Read the model definition and answer for the solid it produces. Units are mm, in the model's axes. A direction names the side the tool comes from. Coordinates: 2 decimals unless noted, no trailing zeros. Loops run counter-clockwise (first coordinate to the right, second up) from the corner with the lowest first, then second, coordinate; pieces in that order, holes last. Notation, with made-up numbers: (83, 10.5) -> (111, 10.5) arc R21 ccw to (111, 23.5) -> close; hole circle Ø11 at (49, 89). An arc over 180 degrees is marked (long way). Answer as CSV lines item,"result".
```python
from build123d import *

# Parameters (mm, degrees)
F0_W     = 5
F0_H     = 3
F1_DEPTH = 5
F2_DEPTH = 23


with BuildPart() as f1:
    # F0 (on Top) → F1 (new body)
    with BuildSketch(Plane.XY):
        Rectangle(F0_W, F0_H)
        with BuildLine():
            ThreePointArc((-0.5, 0.5), (0, 1), (0.5, 0.5))
            Line((0.5, 0.5), (1.27, 0.5))
            ThreePointArc((1.27, 0.5), (1.6235533906, 0.3535533906), (1.77, 0))
            ThreePointArc((1.77, 0), (1.6235533906, -0.3535533906), (1.27, -0.5))
            Line((1.27, -0.5), (0.5, -0.5))
            ThreePointArc((0.5, -0.5), (0, -1), (-0.5, -0.5))
            Line((-0.5, -0.5), (-1.27, -0.5))
            ThreePointArc((-1.27, -0.5), (-1.77, 0), (-1.27, 0.5))
            Line((-1.27, 0.5), (-0.5, 0.5))
        make_face(mode=Mode.SUBTRACT)
        with BuildLine():
            Line((-0.5, 0.5), (0.5, 0.5))
            ThreePointArc((0.5, 0.5), (0, 1), (-0.5, 0.5))
        make_face()
        with BuildLine():
            ThreePointArc((-0.5, 0.5), (-0.3535533906, 0.1464466094), (0, 0))
            ThreePointArc((0, 0), (0.3535533906, 0.1464466094), (0.5, 0.5))
            Line((0.5, 0.5), (-0.5, 0.5))
        make_face()
        with BuildLine():
            ThreePointArc((0.5, -0.5), (0.3535533906, -0.1464466094), (0, 0))
            ThreePointArc((0, 0), (-0.3535533906, -0.1464466094), (-0.5, -0.5))
            Line((-0.5, -0.5), (0.5, -0.5))
        make_face()
        with BuildLine():
            ThreePointArc((-0.5, -0.5), (0, -1), (0.5, -0.5))
            Line((0.5, -0.5), (-0.5, -0.5))
        make_face()
        with BuildLine():
            ThreePointArc((-0.5, -0.5), (-0.3535533906, -0.1464466094), (0, 0))
            ThreePointArc((0, 0), (-0.3535533906, 0.1464466094), (-0.5, 0.5))
            Line((-0.5, 0.5), (-1.27, 0.5))
            ThreePointArc((-1.27, 0.5), (-0.9164466094, 0.3535533906), (-0.77, 0))
            ThreePointArc((-0.77, 0), (-0.9164466094, -0.3535533906), (-1.27, -0.5))
            Line((-1.27, -0.5), (-0.5, -0.5))
        make_face()
        with BuildLine():
            ThreePointArc((0.5, 0.5), (0.3535533906, 0.1464466094), (0, 0))
            Line((0, 0), (0.77, 0))
            ThreePointArc((0.77, 0), (0.9164466094, 0.3535533906), (1.27, 0.5))
            Line((1.27, 0.5), (0.5, 0.5))
        make_face()
        with BuildLine():
            Line((0.77, 0), (0, 0))
            ThreePointArc((0, 0), (0.3535533906, -0.1464466094), (0.5, -0.5))
            Line((0.5, -0.5), (1.27, -0.5))
            ThreePointArc((1.27, -0.5), (0.9164466094, -0.3535533906), (0.77, 0))
        make_face()
    extrude(amount=F1_DEPTH)

    # F0 (on Top) → F2 (join)
    with BuildSketch(Plane.XY):
        with BuildLine():
            ThreePointArc((-0.5, -0.5), (-0.3535533906, -0.1464466094), (0, 0))
            ThreePointArc((0, 0), (-0.3535533906, 0.1464466094), (-0.5, 0.5))
            Line((-0.5, 0.5), (-1.27, 0.5))
            ThreePointArc((-1.27, 0.5), (-0.9164466094, 0.3535533906), (-0.77, 0))
            ThreePointArc((-0.77, 0), (-0.9164466094, -0.3535533906), (-1.27, -0.5))
            Line((-1.27, -0.5), (-0.5, -0.5))
        make_face()
        with BuildLine():
            ThreePointArc((0.5, -0.5), (0.3535533906, -0.1464466094), (0, 0))
            ThreePointArc((0, 0), (-0.3535533906, -0.1464466094), (-0.5, -0.5))
            Line((-0.5, -0.5), (0.5, -0.5))
        make_face()
        with BuildLine():
            ThreePointArc((-0.5, -0.5), (0, -1), (0.5, -0.5))
            Line((0.5, -0.5), (-0.5, -0.5))
        make_face()
        with BuildLine():
            ThreePointArc((-0.5, 0.5), (-0.3535533906, 0.1464466094), (0, 0))
            ThreePointArc((0, 0), (0.3535533906, 0.1464466094), (0.5, 0.5))
            Line((0.5, 0.5), (-0.5, 0.5))
        make_face()
        with BuildLine():
            Line((-0.5, 0.5), (0.5, 0.5))
            ThreePointArc((0.5, 0.5), (0, 1), (-0.5, 0.5))
        make_face()
        with BuildLine():
            ThreePointArc((0.5, 0.5), (0.3535533906, 0.1464466094), (0, 0))
            Line((0, 0), (0.77, 0))
            ThreePointArc((0.77, 0), (0.9164466094, 0.3535533906), (1.27, 0.5))
            Line((1.27, 0.5), (0.5, 0.5))
        make_face()
        with BuildLine():
            Line((0.77, 0), (0, 0))
            ThreePointArc((0, 0), (0.3535533906, -0.1464466094), (0.5, -0.5))
            Line((0.5, -0.5), (1.27, -0.5))
            ThreePointArc((1.27, -0.5), (0.9164466094, -0.3535533906), (0.77, 0))
        make_face()
    extrude(amount=F2_DEPTH)


solid = f1.part
```
Q1. A cutting plane is placed at D-D, the plane y = 0.7. Write down the section's boundary in (x, z).
Results:
outline,"(-2.5, 0) -> (2.5, 0) -> (2.5, 5) -> (0.46, 5) -> (0.46, 23) -> (-0.46, 23) -> (-0.46, 5) -> (-2.5, 5) -> close"
Q2. A cutting plane is placed at A-A, the plane y = -0.3. Write down the section's boundary in (x, z), and give its area (3 significant figures).
Results:
outline,"(-2.5, 0) -> (-1.67, 0) -> (-1.67, 5) -> (-2.5, 5) -> close; (-0.87, 0) -> (0.87, 0) -> (0.87, 23) -> (-0.87, 23) -> close; (1.67, 0) -> (2.5, 0) -> (2.5, 5) -> (1.67, 5) -> close"
area,"48.3 mm²"
Q3. A cutting plane is placed at B-B, the plane z = 3. Write down the section's boundary in (x, y), and give its area (3 significant figures).
Results:
outline,"(-2.5, -1.5) -> (2.5, -1.5) -> (2.5, 1.5) -> (-2.5, 1.5) -> close; hole circle Ø1 at (-1.27, 0); hole circle Ø1 at (1.27, 0)"
area,"13.4 mm²"
Q4. For faces 1 (the face through (0.77, -0.02, 8.78)), 2 (the face through (0, 1, 14)), 3 (the face through (-1, 1, 5)), determine the directions among +Z, -Z, +X, -X, +Y, -Y from which every point of the face is accessible in a straight line to the end or side of a thin tool.
Results:
face 1,"+Z, -Z"
face 2,"+Z, +Y"
face 3,"+Z"
Q5. Given pin 1 Ø1.5 at (x, z) = (1.5, 11) entering from -Y; pin 2 Ø1 at (x, z) = (-1.5, 13.5) entering from +Y, each flat-ended and moving along its own axis, determine where each tip first touches the part or whether it passes through.
Results:
pin 1,"stops at y = -0.5"
pin 2,"stops at y = 0.5"
Q6. Find the intervals of material crossed by probe 1 along X at (y, z) = (0, 10.75); probe 2 along Z at (x, y) = (-1.2, -1); probe 3 along Y at (x, z) = (-0.7, 17.25), in increasing order. Write a range as [from, to].
Results:
probe 1,"x = [-0.77, 0.77]"
probe 2,"z = [0, 5]"
probe 3,"y = [-0.5, 0.5]"
Q7. For a pull along X with two mould halves and no side action, classify faces 4 (the face through (0, -1.5, 2)), 5 (the face through (0, -1, 14)), 6 (the face through (-0.774, -0.065, 8.783)) as pulls with the +X half, pulls with the -X half, needs draft (parallel to the pull), parting line crosses it, or undercut.
Results:
face 4,"needs draft"
face 5,"parting line crosses it"
face 6,"undercut"
Q8. A cutting plane is placed at C-C, the plane z = 15.25. Write down the section's boundary in (x, y), and give its area (3 significant figures).
Results:
outline,"(-1.27, -0.5) -> (-0.5, -0.5) arc R0.5 ccw to (0.5, -0.5) -> (1.27, -0.5) arc R0.5 cw to (1.27, 0.5) -> (0.5, 0.5) arc R0.5 ccw to (-0.5, 0.5) -> (-1.27, 0.5) arc R0.5 cw to start"
area,"2.54 mm²"
